Check sheet for the modelled part. Datum: model origin and axes. Units: mm. A direction names the side the tool comes from. Coordinates: 2 decimals unless noted, no trailing zeros. Write each loop counter-clockwise with the first axis right and the second up, starting at its lowest first coordinate (ties: lowest second). Pieces come first, ordered by that corner, then holes. Notation, with made-up numbers: (8, 78) - (65, 78) arc R27 cw to (65, 113) - close; hole circle Ø2 at (37.25, 71). An arc over 180 degrees is marked (long way). Answer as CSV lines item,"result". Start each with the question number.
from build123d import *

# Parameters (mm, degrees)
SKETCH_1_W      = 26
SKETCH_1_H      = 10.5
SKETCH_1_R      = 1.5
EXTRUDE_1_DEPTH = 95
SKETCH_2_W      = 9
SKETCH_2_H      = 26
EXTRUDE_2_DEPTH = 32
SKETCH_4_R      = 3
EXTRUDE_3_DEPTH = 52
EXTRUDE_START   = 10
SKETCH_4_5_R    = 3
EXTRUDE_4_DEPTH = 10


with BuildPart() as part:
    # 草图1 → 凸台-拉伸1 (new body)
    with BuildSketch(Plane(origin=(0, 0, 0), x_dir=(0, 0, -1), z_dir=(1, 0, 0))):
        with Locations((-13, 5.25)):
            Rectangle(SKETCH_1_W, SKETCH_1_H)
        with Locations((-19.5, 3)):
            Circle(SKETCH_1_R, mode=Mode.SUBTRACT)
        with Locations((-5.5, 3)):
            Circle(SKETCH_1_R, mode=Mode.SUBTRACT)
    extrude(amount=-EXTRUDE_1_DEPTH)

    # 草图2 → 凸台-拉伸2 (add)
    with BuildSketch(Plane(origin=(0, 10.5, 0), x_dir=(1, 0, 0), z_dir=(0, 1, 0))):
        with Locations((-34.5, -13)):
            Rectangle(SKETCH_2_W, SKETCH_2_H)
        with Locations((-86.5, -13)):
            Rectangle(SKETCH_2_W, SKETCH_2_H)
    extrude(amount=EXTRUDE_2_DEPTH)

    # 草图4 → 凸台-拉伸3 (add)
    with BuildSketch(Plane(origin=(-30, 0, 0), x_dir=(0, 0, -1), z_dir=(1, 0, 0))):
        with Locations((-14.5, 24)):
            Circle(SKETCH_4_R)
    extrude(amount=-EXTRUDE_3_DEPTH)

    # 草图4<5> → 凸台-拉伸4 (add)
    with BuildSketch(Plane(origin=(-30, 0, 0), x_dir=(0, 0, -1), z_dir=(1, 0, 0)).offset(EXTRUDE_START)):
        with Locations((-14.5, 24)):
            Circle(SKETCH_4_5_R)
    extrude(amount=-EXTRUDE_4_DEPTH)


solid = part.part
(1) Cross-section at B-B on y = 30.5. Record the boundary of the cut face in (x, z), plus the area to 3 significant figures.
(2) Cross-section at A-A on x = -27.5. Record the boundary of the cut face in (y, z), plus the area to 3 significant figures.
(3) Release check for a two-part mould opening along X. For faces 1 (the face through (-93, 10.5, 13)), 2 (the face through (-60.2, 24.1, 17.5)), 3 (the face through (-95, 5, 13)) record: pulls with the +X half, pulls with the -X half, needs draft (parallel to the pull), parting line crosses it, or undercut.
(4) Material ranges on probe 1 along X at (y, z) = (27, 10); probe 2 along Y at (x, z) = (-21.5, 5.5); probe 3 along Y at (x, z) = (-15, 16.75), recorded low to high. Write a range as from..to.
(5) Cross-section at D-D on y = 3. Record the boundary of the cut face in (x, z).
(6) Cross-section at C-C on z = 5.5. Record the boundary of the cut face in (x, y), plus the area to 3 significant figures.
(7) Tool access check on faces 4 (the face through (-91, 26, 13)), 5 (the face through (-20, 24, 15)), 6 (the face through (-24.9, 24.1, 17.5)). Record the directions out of +Z, -Z, +X, -X, +Y, -Y that give a thin tool (end or side, any length) a straight path to the whole face; none if there is none.
(8) Go/stop test with flat-tipped pins: P1, Ø8, axis at y = 27, z = 12.5, coming from the -X side; P2, Ø12, axis at y = 21.5, z = 15, coming from the +X side; P3, Ø8, axis at x = -57.5, z = 12.5, coming from the +Y side. Record where each tip stops, or that it passes through.
Checked values:
1,outline,"(-91, 0) - (-82, 0) - (-82, 26) - (-91, 26) - close; (-39, 0) - (-30, 0) - (-30, 26) - (-39, 26) - close"
1,area,"468 mm^2"
2,outline,"(0, 0) - (10.5, 0) - (10.5, 26) - (0, 26) - close; circle Ø6 at (24, 14.5); hole circle Ø3 at (3, 5.5); hole circle Ø3 at (3, 19.5)"
2,area,"287 mm^2"
3,face 1,"needs draft"
3,face 2,"undercut"
3,face 3,"pulls with the -X half"
4,probe 1,"-91..-82, -39..-30"
4,probe 2,"0..1.5, 4.5..10.5"
4,probe 3,"0..10.5"
5,outline,"(-95, 0) - (0, 0) - (0, 4) - (-95, 4) - close; (-95, 7) - (0, 7) - (0, 18) - (-95, 18) - close; (-95, 21) - (0, 21) - (0, 26) - (-95, 26) - close"
6,outline,"(-95, 0) - (0, 0) - (0, 1.5) - (-95, 1.5) - close; (-95, 4.5) - (0, 4.5) - (0, 10.5) - (-30, 10.5) - (-30, 42.5) - (-39, 42.5) - (-39, 10.5) - (-82, 10.5) - (-82, 42.5) - (-91, 42.5) - (-91, 10.5) - (-95, 10.5) - close"
6,area,"1,290 mm^2"
7,face 4,"+Z, -Z, -X, +Y"
7,face 5,"+Z, -Z, +X, +Y"
7,face 6,"+X"
8,P1,"x = -91"
8,P2,"x = -20"
8,P3,"y = 27"
